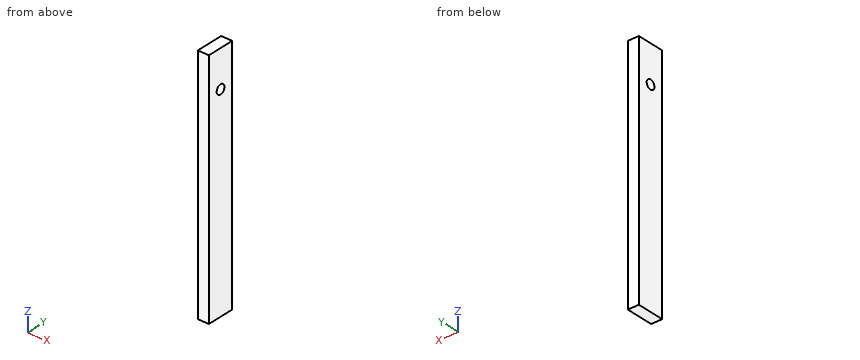
from build123d import *

# Parameters (mm, degrees)
ESQUISSE1_W             = 6
ESQUISSE1_H             = 15
BOSS_EXTRU_1_DEPTH      = 170
ESQUISSE2_R             = 2.5
ENL_V_MAT_EXTRU_1_DEPTH = 10
SKETCH1_W               = 6
SKETCH1_H               = 15
CUT_EXTRUDE1_DEPTH      = 40


with BuildPart() as part:
    # Esquisse1 → Boss.-Extru.1 (new body)
    with BuildSketch(Plane.XY):
        Rectangle(ESQUISSE1_W, ESQUISSE1_H)
    extrude(amount=BOSS_EXTRU_1_DEPTH)

    # Esquisse2 → Enlèv. mat.-Extru.1 (cut)
    with BuildSketch(Plane(origin=(3, 0, 0), x_dir=(0, 0, -1), z_dir=(1, 0, 0))):
        with Locations(Location((-150, 0, 0), (0, 0, 90))):
            Circle(ESQUISSE2_R)
    extrude(amount=-ENL_V_MAT_EXTRU_1_DEPTH, mode=Mode.SUBTRACT)

    # Sketch1 → Cut-Extrude1 (cut)
    with BuildSketch(Plane(origin=(0, 0, 0), x_dir=(-1, 0, 0), z_dir=(0, 0, -1))):
        Rectangle(SKETCH1_W, SKETCH1_H)
    extrude(amount=-CUT_EXTRUDE1_DEPTH, mode=Mode.SUBTRACT)


solid = part.part
The listing builds one solid part. Answer for the finished solid, in the listing's coordinates (mm). Coordinates: 2 decimals unless noted, no trailing zeros. Loops run counter-clockwise (first coordinate to the right, second up) from the corner with the lowest first, then second, coordinate; pieces in that order, holes last.
1) Find section B-B on y = 0. Write down the section's boundary in (x, z).
2) Find the intervals of material crossed by L1, parallel to Z at x = -1.6, y = 0; L2, parallel to Y at x = -1.7, z = 150; L3, parallel to Z at x = -1.45, y = -0.5, in increasing order.
3) Find section A-A on z = 150. Write down the section's boundary in (x, y).
Values:
1. outline: (-3, 40) - (3, 40) - (3, 147.5) - (-3, 147.5) - close; (-3, 152.5) - (3, 152.5) - (3, 170) - (-3, 170) - close
2. L1: z = 40 to 147.5, 152.5 to 170
2. L2: y = -7.5 to -2.5, 2.5 to 7.5
2. L3: z = 40 to 147.55, 152.45 to 170
3. outline: (-3, -7.5) - (3, -7.5) - (3, -2.5) - (-3, -2.5) - close; (-3, 2.5) - (3, 2.5) - (3, 7.5) - (-3, 7.5) - close
